```python
from build123d import *

# Parameters (mm, degrees)
SKETCH1_W           = 115
SKETCH1_H           = 150
BOSS_EXTRUDE1_DEPTH = 3
SKETCH2_W           = 26
SKETCH2_H           = 66
SKETCH2_W_2         = 70.1
SKETCH2_H_2         = 50
CUT_EXTRUDE1_DEPTH  = 3
SKETCH5_W           = 10.3
SKETCH5_H           = 2.3
SKETCH5_W_2         = 2.3
SKETCH5_H_2         = 56.3
CUT_EXTRUDE2_DEPTH  = 3
SKETCH9_W           = 30
SKETCH9_H           = 3
BOSS_EXTRUDE2_DEPTH = 35
SKETCH8_R           = 0.75
SKETCH8_W           = 40
SKETCH8_H           = 40
CUT_EXTRUDE3_DEPTH  = 205.609994868


with BuildPart() as part:
    # Sketch1 → Boss-Extrude1 (new body)
    with BuildSketch(Plane(origin=(0, 0, 0), x_dir=(1, 0, 0), z_dir=(0, 1, 0))):
        Rectangle(SKETCH1_W, SKETCH1_H)
    extrude(amount=-BOSS_EXTRUDE1_DEPTH)

    # Sketch2 → Cut-Extrude1 (cut)
    with BuildSketch(Plane(origin=(0, 0, 0), x_dir=(1, 0, 0), z_dir=(0, 1, 0))):
        with Locations((44.5, -75)):
            Rectangle(SKETCH2_W, SKETCH2_H)
        with Locations((44.5, 75)):
            Rectangle(SKETCH2_W, SKETCH2_H)
        with Locations((-22.45, -50)):
            Rectangle(SKETCH2_W_2, SKETCH2_H_2)
    extrude(amount=-CUT_EXTRUDE1_DEPTH, mode=Mode.SUBTRACT)

    # Sketch5 → Cut-Extrude2 (cut)
    with BuildSketch(Plane.XZ.offset(3)):
        with Locations((32.5, 34)):
            Rectangle(SKETCH5_W, SKETCH5_H)
        with Locations((42.5, 0)):
            Rectangle(SKETCH5_W_2, SKETCH5_H_2)
        with Locations((52.5, 34)):
            Rectangle(SKETCH5_W, SKETCH5_H)
        with Locations((32.5, -34)):
            Rectangle(SKETCH5_W, SKETCH5_H)
        with Locations((52.5, -34)):
            Rectangle(SKETCH5_W, SKETCH5_H)
    extrude(amount=-CUT_EXTRUDE2_DEPTH, mode=Mode.SUBTRACT)

    # Mirror1: part across plane


with BuildPart() as part_1:
    add(part.part)
    add(part.part.mirror(Plane(origin=(-57.5, -3, 75), x_dir=(0, 0, 1), z_dir=(-1, 0, 0))))

    # Sketch9 → Boss-Extrude2 (add)
    with BuildSketch(Plane(origin=(0, 0, -75), x_dir=(-1, 0, 0), z_dir=(0, 0, -1))):
        with Locations((108.7, -1.5)):
            Rectangle(SKETCH9_W, SKETCH9_H)
    extrude(amount=BOSS_EXTRUDE2_DEPTH)

    # Sketch8 → Cut-Extrude3 (cut, through all)
    with BuildSketch(Plane.XZ.offset(3)):
        with Locations(Location((-74.5, -58.832861148, 0), (0, 0, 270))):
            Circle(SKETCH8_R)
        with Locations(Location((-40.5, -58.832861148, 0), (0, 0, 270))):
            Circle(SKETCH8_R)
        with Locations(Location((-104.8, -21.135456144, 0), (0, 0, 270))):
            Circle(SKETCH8_R)
        with Locations(Location((-113.8, -5.135456144, 0), (0, 0, 270))):
            Circle(SKETCH8_R)
        with Locations(Location((-87.980765301, 7.641432582, 0), (0, 0, 270))):
            Circle(SKETCH8_R)
        with Locations(Location((-103.980765301, 16.641432582, 0), (0, 0, 270))):
            Circle(SKETCH8_R)
        with Locations(Location((-104.2, -107, 0), (0, 0, 270))):
            Circle(SKETCH8_R)
        with Locations(Location((-113.2, -91, 0), (0, 0, 270))):
            Circle(SKETCH8_R)
        with Locations((-57.5, 0)):
            Rectangle(SKETCH8_W, SKETCH8_H)
    extrude(amount=-CUT_EXTRUDE3_DEPTH, mode=Mode.SUBTRACT)


solid = part_1.part
```
Part model, mm, in its own coordinate system. Coordinates: 2 decimals unless noted, no trailing zeros. Loops run counter-clockwise (first coordinate to the right, second up) from the corner with the lowest first, then second, coordinate; pieces in that order, holes last. Notation, with made-up numbers: (-32.75, 46) - (23.25, 46) arc R17 ccw to (23.25, 52) - close; hole circle Ø2 at (87, 7). An arc over 180 degrees is marked (long way). Write item = value, one per line. Start each with the question number.
Item 1: Wall check: L1, parallel to Z at x = 29, y = -0.2; L2, parallel to X at y = -2.2, z = 38; L3, parallel to Z at x = -53, y = -2.25. Give the ranges that are in metal, low to high. Write a range as from..to.
Item 2: Flat gauge pins, fed straight in: pin 1 Ø0.9 at (x, z) = (-113.8, -5.14) entering from +Y; pin 2 Ø0.9 at (x, y) = (-65.5, -1) entering from +Z; pin 3 Ø1.2 at (x, y) = (-157, -1) entering from -Z; pin 4 Ø0.7 at (y, z) = (-1.5, 34) entering from -X. Where does each tip first touch, or does it go through?
Item 3: Cut at C-C, the plane y = -1.9. State how many separate pieces and enclosed holes the cut face has, and give its area (3 significant figures).
Item 4: Cut at B-B, the plane z = -65. Give the cut face in (x, y).
Item 5: Cut at D-D, the plane x = 20.5. Give the cut face in (y, z).
Item 6: Cut at A-A, the plane x = -52. Give the cut face in (y, z).
The answers:
q1.L1 = -75..-35.15, -32.85..32.85, 35.15..75
q1.L2 = -172.5..-127.6, 12.6..57.5
q1.L3 = -75..-20, 20..25
q2.pin_1 = through
q2.pin_2 = 25
q2.pin_3 = -42
q2.pin_4 = -162.35
q3.separate_pieces = 1
q3.enclosed_holes = 15
q3.area = 23,000 mm2
q4.outline = (-146.5, -3) - (31.5, -3) - (31.5, 0) - (-146.5, 0) - close
q5.outline = (-3, -75) - (0, -75) - (0, 75) - (-3, 75) - close
q6.outline = (-3, -75) - (0, -75) - (0, -20) - (-3, -20) - close; (-3, 20) - (0, 20) - (0, 25) - (-3, 25) - close
